Read the model definition and answer for the solid it produces. Units are mm, in the model's axes. Face numbers are marked on the shaded views. A direction names the side the tool comes from. Give positions to 0.01 mm unless a question says otherwise; leave off trailing zeros. Write each loop counter-clockwise with the first axis right and the second up, starting at its lowest first coordinate (ties: lowest second). Pieces come first, ordered by that corner, then holes. Notation, with made-up numbers: M 15,-10.5 L 23,-10.5 A3 ccw 23,-6.5 Z; hole C -8,-35 d10. An arc over 180 degrees is marked long. Use a Markdown table: item, result. Add a question column.
Item 1: A cutting plane is placed at D-D on x = 24.2. Determine the outline of the cut face in (y, z), then the cut area to 3 significant figures.
Item 2: A cutting plane is placed at A-A on z = 0. Determine the outline of the cut face in (x, y).
Item 3: Given P1, Ø1.5, axis at x = 9, z = -1.5, coming from the -Y side; P2, Ø1.3, axis at y = -10, z = 3.5, coming from the -X side; P3, Ø12, axis at y = -4.5, z = 0.5, coming from the +X side; P4, Ø9, axis at x = 10, y = 0, coming from the -Z side, each flat-ended and moving along its own axis, determine where each tip first touches the part or whether it passes through.
Item 4: The mould has two halves that part along Y. Classify the marked faces 4, 5 and 6: pulls with the +Y half, pulls with the -Y half, needs draft (parallel to the pull), parting line crosses it, or undercut.
Item 5: A cutting plane is placed at C-C on y = 0. Determine the outline of the cut face in (x, z).
Item 6: For the marked faces 1, 2 and 3, determine the directions among +Z, -Z, +X, -X, +Y, -Y from which every point of the face is accessible in a straight line to the end or side of a thin tool.
Item 7: A cutting plane is placed at B-B on x = 10. Determine the outline of the cut face in (y, z), then the cut area to 3 significant figures.
Item 8: Consider probe 1 along X at (y, z) = (0.25, -1); probe 2 along X at (y, z) = (7.75, 0); probe 3 along Z at (x, y) = (32.5, -7.25). Determine where each line is inside the solid, lowest interval first. Write a range as [from, to].
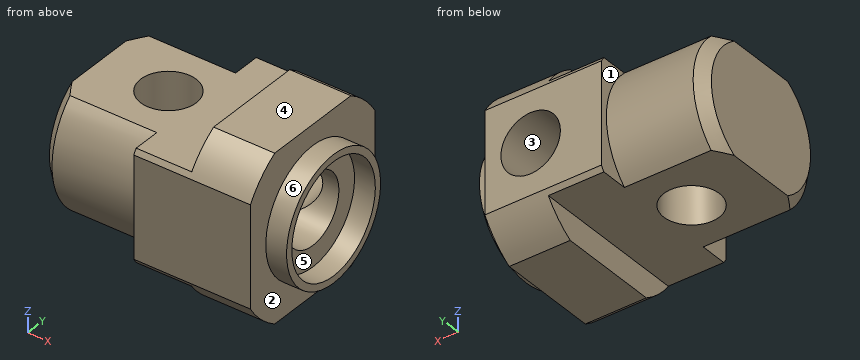
from build123d import *

# Parameters (mm, degrees)
CROQUIS2_OUTSIDE_W      = 40.034
CROQUIS2_OUTSIDE_H      = 40.034
CROQUIS2_OUTSIDE_W_2    = 23.9
CROQUIS2_OUTSIDE_H_2    = 23.9
CORTAR_EXTRUIR1_DEPTH   = 37.614751126
CROQUIS3_OUTSIDE_W      = 35.046
CROQUIS3_OUTSIDE_H      = 35.046
CROQUIS3_OUTSIDE_W_2    = 16
CROQUIS3_OUTSIDE_H_2    = 32
CORTAR_EXTRUIR2_DEPTH   = 22
CROQUIS4_R              = 9
CROQUIS4_R_2            = 8
SALIENTE_EXTRUIR1_DEPTH = 3
CROQUIS5_R              = 4
CORTAR_EXTRUIR3_DEPTH   = 42.027368914
CROQUIS8_R              = 5
CORTAR_EXTRUIR4_DEPTH   = 13
CROQUIS7_R              = 4.283
CORTAR_EXTRUIR5_DEPTH   = 13


with BuildPart() as part:
    # Croquis1 → Revolución1 (revolve)
    with BuildSketch(Plane(origin=(0, 0, 0), x_dir=(1, 0, 0), z_dir=(0, 1, 0)), mode=Mode.PRIVATE) as revoluci_n1_sk:
        Polygon((0, 0), (30.8, 0), (30.8, 14), (14, 14), (14, 11), (1.5, 11), (0, 9.5), align=None)
    revolve(revoluci_n1_sk.sketch.rotate(Axis((0, 0, 0), (1, 0, 0)), 180), axis=Axis((0, 0, 0), (1, 0, 0)))

    # Croquis2 outside → Cortar-Extruir1 (cut, through all)
    with BuildSketch(Plane(origin=(0, 0, 0), x_dir=(0, 0, -1), z_dir=(1, 0, 0))):
        Rectangle(CROQUIS2_OUTSIDE_W, CROQUIS2_OUTSIDE_H)
        Rectangle(CROQUIS2_OUTSIDE_W_2, CROQUIS2_OUTSIDE_H_2, mode=Mode.SUBTRACT)
    extrude(amount=CORTAR_EXTRUIR1_DEPTH, mode=Mode.SUBTRACT)

    # Croquis3 outside → Cortar-Extruir2 (cut)
    with BuildSketch(Plane(origin=(0, 0, 0), x_dir=(0, 0, -1), z_dir=(1, 0, 0))):
        Rectangle(CROQUIS3_OUTSIDE_W, CROQUIS3_OUTSIDE_H)
        Rectangle(CROQUIS3_OUTSIDE_W_2, CROQUIS3_OUTSIDE_H_2, mode=Mode.SUBTRACT)
    extrude(amount=CORTAR_EXTRUIR2_DEPTH, mode=Mode.SUBTRACT)

    # Croquis4 → Saliente-Extruir1 (add)
    with BuildSketch(Plane(origin=(30.8, 0, 0), x_dir=(0, 0, -1), z_dir=(1, 0, 0))):
        with Locations(Location((0, 0, 0), (0, 0, 180))):
            Circle(CROQUIS4_R)
        Circle(CROQUIS4_R_2, mode=Mode.SUBTRACT)
    extrude(amount=SALIENTE_EXTRUIR1_DEPTH)

    # Croquis5 → Cortar-Extruir3 (cut, through all)
    with BuildSketch(Plane.XY.offset(8)):
        with Locations((10, 0)):
            Circle(CROQUIS5_R)
    extrude(amount=-CORTAR_EXTRUIR3_DEPTH, mode=Mode.SUBTRACT)

    # Croquis8 → Cortar-Extruir4 (cut)
    with BuildSketch(Plane(origin=(30.8, 0, 0), x_dir=(0, 0, -1), z_dir=(1, 0, 0))):
        Circle(CROQUIS8_R)
    extrude(amount=-CORTAR_EXTRUIR4_DEPTH, mode=Mode.SUBTRACT)

    # Croquis7 → Cortar-Extruir5 (cut)
    with BuildSketch(Plane(origin=(0, 11.95, 0), x_dir=(1, 0, 0), z_dir=(0, 1, 0))):
        with Locations(Location((24.2, 0, 0), (0, 0, 270))):
            Circle(CROQUIS7_R)
    extrude(amount=-CORTAR_EXTRUIR5_DEPTH, mode=Mode.SUBTRACT)


solid = part.part
Filled in:
| question | item | result |
|---|---|---|
| 1 | outline | M -11.95,-7.29 A14 ccw -7.29,-11.95 L 7.29,-11.95 A14 ccw 11.95,-7.29 L 11.95,-4.28 L 2.58,-4.28 A5 cw long 2.58,4.28 L 11.95,4.28 L 11.95,7.29 A14 ccw 7.29,11.95 L -7.29,11.95 A14 ccw -11.95,7.29 Z |
| 1 | area | 391 mm² |
| 2 | outline | M 0,-9.5 L 1.5,-11 L 14,-11 L 14,-11.95 L 30.8,-11.95 L 30.8,-9 L 33.8,-9 L 33.8,-8 L 30.8,-8 L 30.8,-5 L 17.8,-5 L 17.8,5 L 19.92,5 L 19.92,11.95 L 14,11.95 L 14,11 L 1.5,11 L 0,9.5 Z; M 28.48,5 L 30.8,5 L 30.8,8 L 33.8,8 L 33.8,9 L 30.8,9 L 30.8,11.95 L 28.48,11.95 Z; hole C 10,0 d8 |
| 3 | P1 | y = -10.97 |
| 3 | P2 | x = 0.44 |
| 3 | P3 | x = 33.8 |
| 3 | P4 | z = -8 |
| 4 | face 4 | needs draft |
| 4 | face 5 | undercut |
| 4 | face 6 | parting line crosses it |
| 5 | outline | M 0,-8 L 6,-8 L 6,8 L 0,8 Z; M 14,-8 L 22,-8 L 22,-11.95 L 30.8,-11.95 L 30.8,-9 L 33.8,-9 L 33.8,-8 L 30.8,-8 L 30.8,-5 L 17.8,-5 L 17.8,5 L 30.8,5 L 30.8,8 L 33.8,8 L 33.8,9 L 30.8,9 L 30.8,11.95 L 22,11.95 L 22,8 L 14,8 Z |
| 6 | face 1 | -X, +Y |
| 6 | face 2 | +X |
| 6 | face 3 | +Y |
| 7 | outline | M -7.55,-8 L -4,-8 L -4,8 L -7.55,8 A11 ccw Z; M 4,-8 L 7.55,-8 A11 ccw 7.55,8 L 4,8 Z |
| 7 | area | 190 mm² |
| 8 | probe 1 | [0, 6.01], [13.99, 17.8] |
| 8 | probe 2 | [0, 19.92], [28.48, 30.8] |
| 8 | probe 3 | [-5.33, -3.38], [3.38, 5.33] |
